```python
from build123d import *

# Parameters (mm, degrees)
F0_R          = 9
F1_DEPTH      = 13
F2_R          = 2.5
F3_DEPTH      = 13.001
F5_W          = 0.6
F5_H          = 13
F7_DEPTH      = 1.5050013897
F7_DEPTH_BACK = 1.5050013897


with BuildPart() as f1:
    # F0 (on Top) → F1 (new body)
    with BuildSketch(Plane.XY):
        Circle(F0_R)
    extrude(amount=F1_DEPTH)

    # F2 (on face) → F3 (cut, through all)
    with BuildSketch(Plane.XY.offset(13)):
        Circle(F2_R)
    extrude(amount=-F3_DEPTH, mode=Mode.SUBTRACT)


with BuildPart() as f6_1:
    # F6: instance of F1
    add(f1.part.mirror(Plane.XZ.offset(9.5)))


with BuildPart() as f1_1:
    add(f1.part)

    add(f6_1.part)  # F7 merges F6_1
    # F5 (on offset) → F7 (join, two sides)
    with BuildSketch(Plane.XZ.offset(9.5)) as f7_sk:
        with Locations((0, 6.5)):
            Rectangle(F5_W, F5_H)
    extrude(amount=F7_DEPTH)
    extrude(f7_sk.sketch, amount=-F7_DEPTH_BACK)


solid = f1_1.part
```
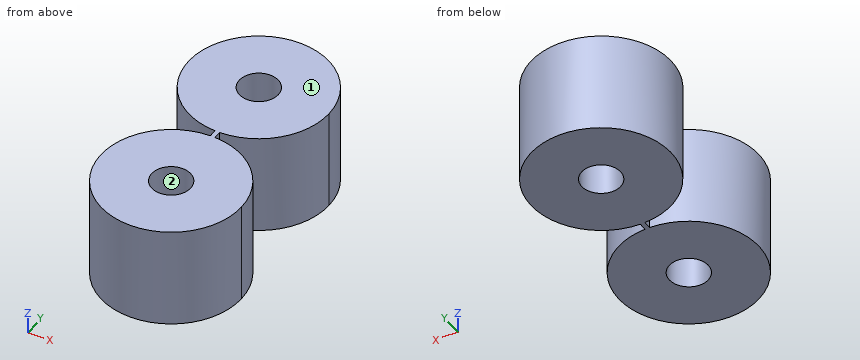
Could you check a few things on this model? Use its own coordinates, in mm. Face numbers are marked on the shaded views. Round coordinates to 2 decimals unless told otherwise and drop trailing zeros. Write each loop counter-clockwise with the first axis right and the second up, starting at its lowest first coordinate (ties: lowest second). Pieces come first, ordered by that corner, then holes.
(1) For pin 1 (3 mm diameter, centred on y = -4.5, z = 2, fed in from +X); pin 2 (0.8 mm diameter, centred on y = -9.5, z = 9.5, fed in from +X); pin 3 (2 mm diameter, centred on x = -1, y = -3, fed in from -Z); pin 4 (4 mm diameter, centred on x = 0, y = 0, fed in from -Z), each with a flat end and sliding along its axis, tell me the tip position at first contact or that it passes through.
Findings below:
pin 1: stops at x = 8.49
pin 2: stops at x = 0.3
pin 3: stops at z = 0
pin 4: passes through
(2) Suppose I cut it at D-D on y = -24.5. Write out the boundary of the cut face in (x, z), and give its area (3 significant figures).
Findings below:
outline: (-7.12, 0) - (7.12, 0) - (7.12, 13) - (-7.12, 13) - close
area: 185 mm2
(3) If I drill on probe 1 along Y at (x, z) = (0, 5); probe 2 along X at (y, z) = (-19, 6); probe 3 along X at (y, z) = (-21, 6), over which ranges is the centre line in solid material (lowest first)?
Findings below:
probe 1: y = -28 to -21.5, -16.5 to -2.5, 2.5 to 9
probe 2: x = -9 to -2.5, 2.5 to 9
probe 3: x = -8.77 to -1.5, 1.5 to 8.77
(4) Thinking about a two-plate mould opening in X: for the marked faces 1 and 2, which applies, +X half, -X half, draft (parallel to the pull), parting line (faces both ways), or undercut?
Findings below:
face 1: draft
face 2: undercut
(5) Suppose I cut it at A-A on x = -3.5. Write out the boundary of the cut face in (y, z), and give its area (3 significant figures).
Findings below:
outline: (-27.29, 0) - (-10.71, 0) - (-10.71, 13) - (-27.29, 13) - close; (-8.29, 0) - (8.29, 0) - (8.29, 13) - (-8.29, 13) - close
area: 431 mm2
(6) Suppose I cut it at B-B on y = 2. Write out the boundary of the cut face in (x, z).
Findings below:
outline: (-8.77, 0) - (-1.5, 0) - (-1.5, 13) - (-8.77, 13) - close; (1.5, 0) - (8.77, 0) - (8.77, 13) - (1.5, 13) - close
(7) Suppose I cut it at C-C on z = 5.5. Write out the boundary of the cut face in (x, y) (3 decimals).
Findings below:
outline: (-0.3, -10.005) arc R9 ccw (long way) to (0.3, -10.005) - (0.3, -8.995) arc R9 ccw (long way) to (-0.3, -8.995) - close; hole circle Ø5 at (0, -19); hole circle Ø5 at (0, 0)
